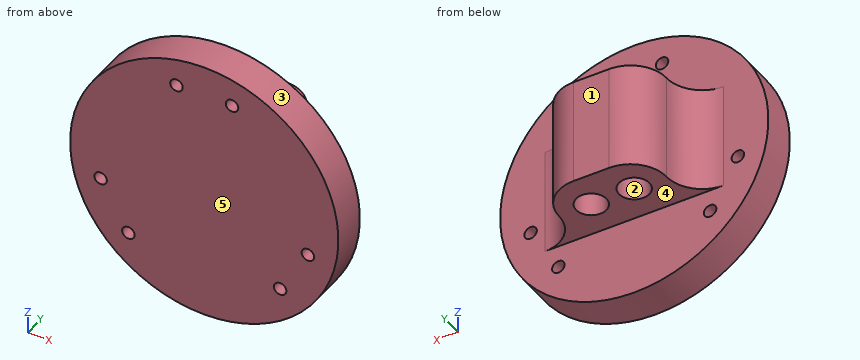
from build123d import *

# Parameters (mm, degrees)
SKETCH1_R           = 37.5
BOSS_EXTRUDE1_DEPTH = 10
SKETCH9_R           = 1.75
CUT_EXTRUDE5_DEPTH  = 54.967582862
CIRPATTERN3_COUNT   = 3
SKETCH10_W          = 30
SKETCH10_H          = 30
BOSS_EXTRUDE2_DEPTH = 20
SKETCH11_R          = 4.25
CUT_EXTRUDE6_DEPTH  = 72.151247354
FILLET1_START       = -15
FILLET1_DEPTH       = 30
FILLET1_2_DEPTH     = 30


with BuildPart() as part:
    # Sketch1 → Boss-Extrude1 (new body)
    with BuildSketch(Plane(origin=(0, 0, 0), x_dir=(1, 0, 0), z_dir=(0, 1, 0))):
        with Locations(Location((0, 0, 0), (0, 0, 270))):
            Circle(SKETCH1_R)
    extrude(amount=BOSS_EXTRUDE1_DEPTH)

    # Sketch9 → Cut-Extrude5 (cut, through all)
    with BuildSketch(Plane(origin=(0, 10, 0), x_dir=(1, 0, 0), z_dir=(0, 1, 0))):
        with Locations(Location((21.213203436, 21.213203436, 0), (0, 0, 270))):
            Circle(SKETCH9_R)
        with Locations(Location((28.977774789, 7.764571353, 0), (0, 0, 270))):
            Circle(SKETCH9_R)
    cut_extrude5 = extrude(amount=-CUT_EXTRUDE5_DEPTH, mode=Mode.SUBTRACT)

    # CirPattern3: Cut-Extrude5 ×3 about axis
    cirpattern3_axis = Axis((0, 0, 0), (0, 1, 0))
    for i in range(1, CIRPATTERN3_COUNT):
        add(cut_extrude5.rotate(cirpattern3_axis, i * 360 / CIRPATTERN3_COUNT), mode=Mode.SUBTRACT)

    # Sketch10 → Boss-Extrude2 (add)
    with BuildSketch(Plane(origin=(0, 10, 0), x_dir=(1, 0, 0), z_dir=(0, 1, 0))):
        Rectangle(SKETCH10_W, SKETCH10_H)
    extrude(amount=BOSS_EXTRUDE2_DEPTH)

    # Sketch11 → Cut-Extrude6 (cut, through all)
    with BuildSketch(Plane.XY.offset(-15)):
        with Locations(Location((6, 20, 0), (0, 0, 180))):
            Circle(SKETCH11_R)
        with Locations(Location((-6, 20, 0), (0, 0, 180))):
            Circle(SKETCH11_R)
    extrude(amount=CUT_EXTRUDE6_DEPTH, mode=Mode.SUBTRACT)

    # Fillet1: read off the stored shape, not the designer's step
    # Fillet1 outline → Fillet1 (cut)
    with BuildSketch(Plane.XY.offset(FILLET1_START)):
        with BuildLine():
            ThreePointArc((5, 30), (12.071067812, 27.071067812), (15, 20))
            Line((15, 20), (15, 30))
            Line((15, 30), (5, 30))
        make_face()
        with BuildLine():
            ThreePointArc((-15, 20), (-12.071067812, 27.071067812), (-5, 30))
            Line((-5, 30), (-15, 30))
            Line((-15, 30), (-15, 20))
        make_face()
    extrude(amount=FILLET1_DEPTH, mode=Mode.SUBTRACT)

    # Fillet1 2 outline → Fillet1 2 (add)
    with BuildSketch(Plane.XY.offset(FILLET1_START)):
        with BuildLine():
            ThreePointArc((25, 10), (17.928932188, 12.928932188), (15, 20))
            Line((15, 20), (15, 10))
            Line((15, 10), (25, 10))
        make_face()
        with BuildLine():
            Line((-25, 10), (-15, 10))
            Line((-15, 10), (-15, 20))
            ThreePointArc((-15, 20), (-17.928932188, 12.928932188), (-25, 10))
        make_face()
    extrude(amount=FILLET1_2_DEPTH)


solid = part.part
Can you work these out from the model? Positions are in its coordinate system, mm. Face numbers are marked on the shaded views. A direction names the side the tool comes from. Give positions to 0.01 mm unless a question says otherwise; leave off trailing zeros. Loops run counter-clockwise (first coordinate to the right, second up) from the corner with the lowest first, then second, coordinate; pieces in that order, holes last. Notation, with made-up numbers: (84, 77.5) - (128, 77.5) arc R29 cw to (128, 106.5) - close; hole circle Ø4 at (38, 7.25). An arc over 180 degrees is marked (long way). Answer as a JSON object with one key per item and string values.
Q1. If we mould it in two halves opening along Y, with no side actions, what happens to the marked faces 1, 2 and 3? For each: pulls with the +Y half, pulls with the -Y half, needs draft (parallel to the pull), parting line crosses it, or undercut.
Geometry says:
{"face 1": "pulls with the +Y half", "face 2": "undercut", "face 3": "needs draft"}
Q2. If I drill on L1, parallel to X at y = 21.5, z = 13.5; L2, parallel to Y at x = 0.5, z = -31.5; L3, parallel to Z at x = 6, y = 25.5, over which ranges is the centre line in solid material (lowest first)?
Geometry says:
{"L1": "-14.89 to -9.98, -2.02 to 2.02, 9.98 to 14.89", "L2": "0 to 10", "L3": "-15 to 15"}
Q3. Imagine slicing it at A-A on z = 0. Write out the boundary of the cut face in (x, y), plus the area to 3 significant figures.
Geometry says:
{"outline": "(-37.5, 0) - (37.5, 0) - (37.5, 10) - (25, 10) arc R10 cw to (15, 20) arc R10 ccw to (5, 30) - (-5, 30) arc R10 ccw to (-15, 20) arc R10 cw to (-25, 10) - (-37.5, 10) - close; hole circle Ø8.5 at (-6, 20); hole circle Ø8.5 at (6, 20)", "area": "1,240 mm²"}
Q4. Imagine slicing it at D-D on x = 8.5. Write out the boundary of the cut face in (y, z), plus the area to 3 significant figures.
Geometry says:
{"outline": "(0, -36.52) - (10, -36.52) - (10, -15) - (16.56, -15) - (16.56, 15) - (10, 15) - (10, 27.39) - (0, 27.39) - close; (0, 30.57) - (10, 30.57) - (10, 36.52) - (0, 36.52) - close; (23.44, -15) - (29.37, -15) - (29.37, 15) - (23.44, 15) - close", "area": "1,070 mm²"}
Q5. Which directions (+Z, -Z, +X, -X, +Y, -Y) give clear straight access to the entire face, cutting with the end or side of a thin tool? Please do the marked faces 4 and 5.
Geometry says:
{"face 4": "-Z, +X, -X, +Y", "face 5": "+Z, -Z, +X, -X, -Y"}
Q6. Imagine slicing it at C-C on y = 21.5. Write out the boundary of the cut face in (x, z), plus the area to 3 significant figures.
Geometry says:
{"outline": "(-14.89, -15) - (-9.98, -15) - (-9.98, 15) - (-14.89, 15) - close; (-2.02, -15) - (2.02, -15) - (2.02, 15) - (-2.02, 15) - close; (9.98, -15) - (14.89, -15) - (14.89, 15) - (9.98, 15) - close", "area": "416 mm²"}
Q7. Imagine slicing it at B-B on x = -21.5. Write out the boundary of the cut face in (y, z).
Geometry says:
{"outline": "(0, -30.72) - (10, -30.72) - (10, -22.94) - (0, -22.94) - close; (0, -19.49) - (10, -19.49) - (10, -15) - (10.63, -15) - (10.63, 15) - (10, 15) - (10, 30.72) - (0, 30.72) - close"}
Q8. Will these pins go through, and if not, where does the flat tip stop? P1, Ø4, axis at y = 10.5, z = -21.5, coming from the +X side; P2, Ø11, axis at x = 6, y = 20, coming from the -Z side; P3, Ø1.5, axis at y = 20, z = 10.5, coming from the -X side.
Geometry says:
{"P1": "x = 31.99", "P2": "z = -15", "P3": "x = -15.03"}
